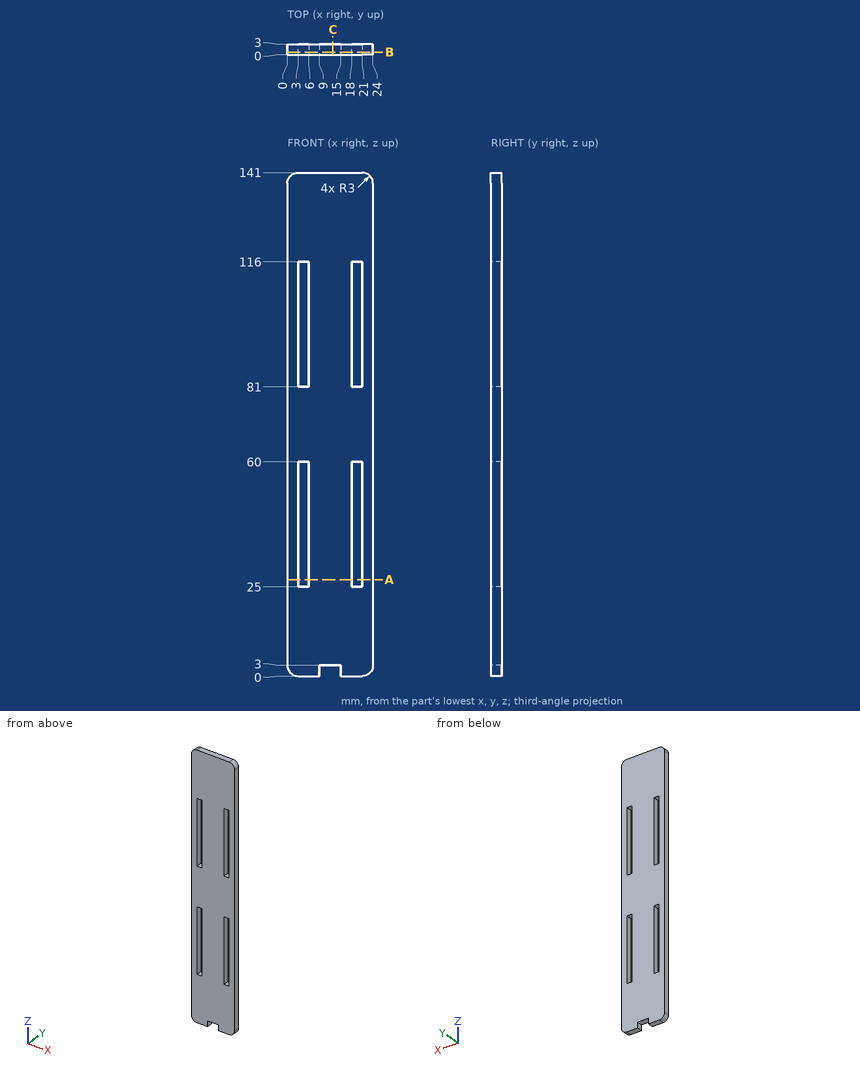
Part print with two shaded views. Sizes in mm from the minimum x, y, z corner. Give positions to 0.01 mm unless a question says otherwise; leave off trailing zeros. Order: outer loops, then holes, each group sorted by start corner. A loop starts at its lowest first (then second) coordinate and runs counter-clockwise, first axis right, second up.
1) Pin check, flat tips, straight feed: pin 1 (0.9 mm diameter, centred on y = 1.5, z = 1.5, fed in from +X); pin 2 (1.5 mm diameter, centred on y = 1.5, z = 1.5, fed in from -X). Stop position of each tip, or through.
2) Saw through at A-A, the plane z = 27. Write the cut outline in (x, y), then the cut area to 3 significant figures.
3) Saw through at C-C, the plane x = 12.75. Write the cut outline in (y, z).
4) Saw through at B-B, the plane y = 0.75. Write the cut outline in (x, z).
5) Wall check: probe 1 along X at (y, z) = (0.5, 49.5); probe 2 along Z at (x, y) = (4, 1.8); probe 3 along Z at (x, y) = (14.25, 0.85). Give the ranges that are in metal, low to high.
Computed:
1. pin 1: stops at x = 23.81
1. pin 2: stops at x = 0.1
2. outline: (0, 0) - (3, 0) - (3, 3) - (0, 3) - close; (6, 0) - (18, 0) - (18, 3) - (6, 3) - close; (21, 0) - (24, 0) - (24, 3) - (21, 3) - close
2. area: 54.0 mm2
3. outline: (0, 3) - (3, 3) - (3, 141) - (0, 141) - close
4. outline: (0, 3) arc R3 ccw to (3, 0) - (9, 0) - (9, 3) - (15, 3) - (15, 0) - (21, 0) arc R3 ccw to (24, 3) - (24, 138) arc R3 ccw to (21, 141) - (3, 141) arc R3 ccw to (0, 138) - close; hole (3, 25) - (6, 25) - (6, 60) - (3, 60) - close; hole (3, 81) - (6, 81) - (6, 116) - (3, 116) - close; hole (18, 25) - (21, 25) - (21, 60) - (18, 60) - close; hole (18, 81) - (21, 81) - (21, 116) - (18, 116) - close
5. probe 1: x = 0 to 3, 6 to 18, 21 to 24
5. probe 2: z = 0 to 25, 60 to 81, 116 to 141
5. probe 3: z = 3 to 141
